```python
from build123d import *

# Parameters (mm, degrees)
SKETCH1_R               = 1.1
BOSS_EXTRUDE1_DEPTH     = 4
SKETCH2_R               = 5.875
BOSS_EXTRUDE2_DEPTH     = 13
CUT_EXTRUDE1_DEPTH      = 49.674942219
CUT_EXTRUDE1_DEPTH_BACK = 49.674942219
SKETCH3_R               = 3.875


with BuildPart() as part:
    # Sketch1 → Boss-Extrude1 (new body)
    with BuildSketch(Plane.XY):
        with BuildLine():
            Line((-4.959780557, 40.132911392), (-9.919561113, 1.265822785))
            ThreePointArc((-9.919561113, 1.265822785), (0, -10), (9.919561113, 1.265822785))
            Line((9.919561113, 1.265822785), (4.959780557, 40.132911392))
            ThreePointArc((4.959780557, 40.132911392), (0, 44.5), (-4.959780557, 40.132911392))
        make_face()
        with Locations((0, 39.5)):
            Circle(SKETCH1_R, mode=Mode.SUBTRACT)
        with Locations((0, 34.5)):
            Circle(SKETCH1_R, mode=Mode.SUBTRACT)
        with Locations((0, 29.5)):
            Circle(SKETCH1_R, mode=Mode.SUBTRACT)
        with Locations((0, 24.5)):
            Circle(SKETCH1_R, mode=Mode.SUBTRACT)
        with Locations((0, 19.5)):
            Circle(SKETCH1_R, mode=Mode.SUBTRACT)
        with Locations((0, 14.5)):
            Circle(SKETCH1_R, mode=Mode.SUBTRACT)
    extrude(amount=BOSS_EXTRUDE1_DEPTH)

    # Sketch2 → Boss-Extrude2 (add)
    with BuildSketch(Plane.XY.offset(4)):
        with Locations(Location((0, 0, 0), (0, 0, 180))):
            Circle(SKETCH2_R)
    extrude(amount=BOSS_EXTRUDE2_DEPTH)

    # Sketch3 → Cut-Extrude1 (cut, two sides: drawn at the far end of the back side and taken through both)
    with BuildSketch(Plane.XY.offset(-CUT_EXTRUDE1_DEPTH_BACK)):
        Circle(SKETCH3_R)
    extrude(amount=CUT_EXTRUDE1_DEPTH + CUT_EXTRUDE1_DEPTH_BACK, mode=Mode.SUBTRACT)


solid = part.part
```
Build history of the part. All positions in model axes, mm. A direction names the side the tool comes from. Coordinates: 2 decimals unless noted, no trailing zeros. Order: outer loops, then holes, each group sorted by start corner. A loop starts at its lowest first (then second) coordinate and runs counter-clockwise, first axis right, second up. Notation, with made-up numbers: (5, -24) -> (34, -24) arc R13 ccw to (34, -19) -> close; hole circle Ø3 at (41.25, 34). An arc over 180 degrees is marked (long way). Answer in a Markdown table with one row per item. Add a question column.
Q1. Mould opens along Y. For faces 1 (the face through (0, 18, 4)), 2 (the face through (7.474, 20.427, 1.972)), 3 (the face through (0.59, 40.43, 1.97)), 4 (the face through (-0.238, 13.426, 1.972)) say: +Y half, -Y half, draft (parallel to the pull), parting line (faces both ways), or undercut.
Q2. Wall check: line 1 along Y through (x, z) = (0, 12) (3 decimals); line 2 along Z through (x, y) = (2, 20.5); line 3 along X through (y, z) = (3, 4.75). Give the ranges that are in metal, low to high. Write a range as [from, to].
Q3. Which spindle directions (+Z, -Z, +X, -X, +Y, -Y) get a long thin tool onto all of the face, cutting with end or side? Do faces 5 (the face through (0.765, -5.825, 10.409)), 6 (the face through (-7.4, 21, 2)). Say none if no direction does.
Q4. Band-saw the part on C-C, the plane z = 7.5. List the corners of the cut face in (x, y) (3 decimals), then the cut area to 3 significant figures.
Q5. Drop flat-ended pins along their axis: pin 1 (8 mm diameter, centred on x = 8, z = 10.5, fed in from +Y); pin 2 (1 mm diameter, centred on x = 0.5, z = 11, fed in from -Y) (3 decimals); pin 3 (9 mm diameter, centred on x = 0, y = 0, fed in from -Z); pin 4 (4 mm diameter, centred on x = -4, z = 8.5, fed in from -Y). Give the stop position or say it passes through.
Q6. Band-saw the part on A-A, the plane y = 29. List the corners of the cut face in (x, z), then the cut area to 3 significant figures.
Q7. Band-saw the part on D-D, the plane y = 14.5. List the corners of the cut face in (x, z), then the cut area to 3 significant figures.
Q8. Band-saw the part on B-B, the plane x = -2. List the corners of the cut face in (y, z).
Answers follow:
| question | item | result |
|---|---|---|
| 1 | face 1 | draft |
| 1 | face 2 | +Y half |
| 1 | face 3 | undercut |
| 1 | face 4 | undercut |
| 2 | line 1 | [-5.875, -3.875], [3.875, 5.875] |
| 2 | line 2 | [0, 4] |
| 2 | line 3 | [-5.05, -2.45], [2.45, 5.05] |
| 3 | face 5 | +Z |
| 3 | face 6 | +Z, -Z, -X, +Y |
| 4 | outline | circle Ø11.75 at (0, 0); hole circle Ø7.75 at (0, 0) |
| 4 | area | 61.3 mm^2 |
| 5 | pin 1 | y = 4.3 |
| 5 | pin 2 | y = -5.875 |
| 5 | pin 3 | z = 0 |
| 5 | pin 4 | y = -5.52 |
| 6 | outline | (-6.38, 0) -> (-0.98, 0) -> (-0.98, 4) -> (-6.38, 4) -> close; (0.98, 0) -> (6.38, 0) -> (6.38, 4) -> (0.98, 4) -> close |
| 6 | area | 43.2 mm^2 |
| 7 | outline | (-8.23, 0) -> (-1.1, 0) -> (-1.1, 4) -> (-8.23, 4) -> close; (1.1, 0) -> (8.23, 0) -> (8.23, 4) -> (1.1, 4) -> close |
| 7 | area | 57.0 mm^2 |
| 8 | outline | (-9.8, 0) -> (-3.32, 0) -> (-3.32, 17) -> (-5.52, 17) -> (-5.52, 4) -> (-9.8, 4) -> close; (3.32, 0) -> (44.08, 0) -> (44.08, 4) -> (5.52, 4) -> (5.52, 17) -> (3.32, 17) -> close |
